Answer from the drawing. Dimensions are ordinates in mm from the lowest x, y and z of the part. Round coordinates to 2 decimals unless told otherwise and drop trailing zeros. Order: outer loops, then holes, each group sorted by start corner. A loop starts at its lowest first (then second) coordinate and runs counter-clockwise, first axis right, second up. Notation, with made-up numbers: M -36,45 L -10,45 A33 ccw -10,81 Z; hole C -25.5,-30 d4. An arc over 180 degrees is marked long. Answer as a JSON object with one key per item and string values. Group by question number.
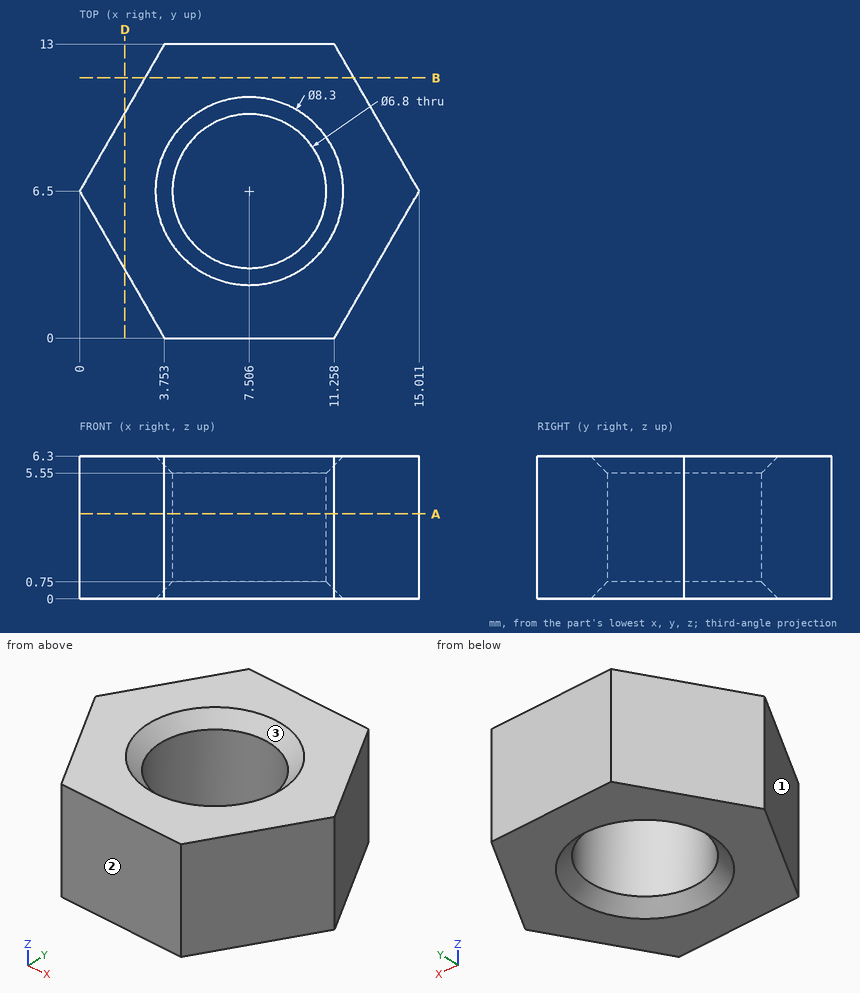
Item 1: This flat-tipped pin is pushed along its axis until it touches: pin 1 (2 mm diameter, centred on y = 3, z = 2.5, fed in from -X). Where does it stop, or does it pass through?
Item 2: Find section D-D (x = 2). Give the vertices of the cut face in (y, z) (1 decimal).
Item 3: Find section B-B (y = 11.5). Give the vertices of the cut face in (x, z) (1 decimal).
Item 4: Find section A-A (z = 3.75). Give the vertices of the cut face in (x, y) (1 decimal).
Item 5: The mould has two halves that part along X. Classify the marked faces 1, 2 and 3: +X half, -X half, draft (parallel to the pull), parting line (faces both ways), or undercut.
Item 6: Consider L1, parallel to Y at x = 8.5, z = 3.25; L2, parallel to X at y = 7, z = 1.25. Determine where each line is inside the solid, lowest interval first.
Responses:
{
 "1": {"pin 1": "stops at x = 1.44"},
 "2": {"outline": "M 3,0 L 10,0 L 10,6.3 L 3,6.3 Z"},
 "3": {"outline": "M 2.9,0 L 12.1,0 L 12.1,6.3 L 2.9,6.3 Z"},
 "4": {"outline": "M 0,6.5 L 3.8,0 L 11.3,0 L 15,6.5 L 11.3,13 L 3.8,13 Z; hole C 7.5,6.5 d6.8"},
 "5": {"face 1": "-X half", "face 2": "draft", "face 3": "undercut"},
 "6": {"L1": "y = 0 to 3.25, 9.75 to 13", "L2": "x = 0.29 to 4.14, 10.87 to 14.72"}
}
